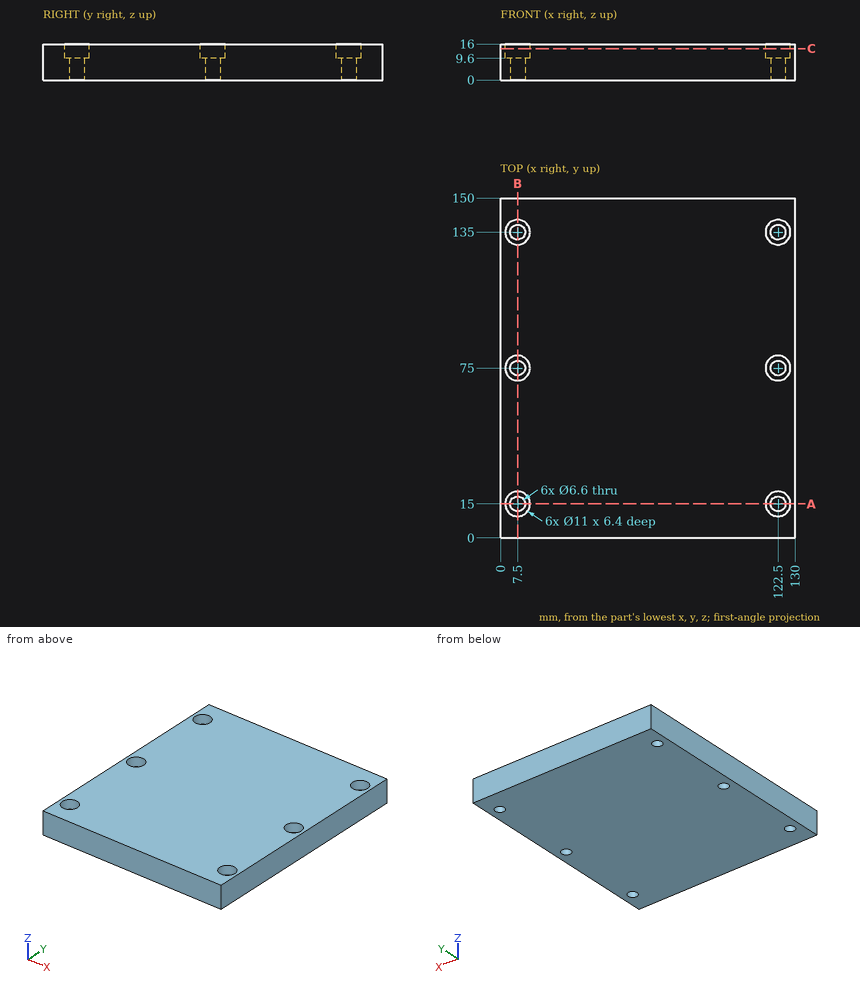
Can you work these out from the drawing? Everything is in mm from the part's minimum corner. Coordinates: 2 decimals unless noted, no trailing zeros. Order: outer loops, then holes, each group sorted by start corner. A loop starts at its lowest first (then second) coordinate and runs counter-clockwise, first axis right, second up. Notation, with made-up numbers: (52, 87) -> (107, 87) arc R18 cw to (107, 105) -> close; hole circle Ø9 at (68, -29). An arc over 180 degrees is marked (long way). Use one line per item in the form item = value.
Q1. I need wall thicknesses on L1, parallel to X at y = 135, z = 6.25; L2, parallel to Y at x = 7.5, z = 13; L3, parallel to X at y = 135, z = 14.75. Which ranges of each line are inside material? Lowest first, please.
From the geometry:
L1 = 0 to 4.2, 10.8 to 119.2, 125.8 to 130
L2 = 0 to 9.5, 20.5 to 69.5, 80.5 to 129.5, 140.5 to 150
L3 = 0 to 2, 13 to 117, 128 to 130
Q2. Imagine slicing it at C-C, the plane z = 14. List the corners of the cut face in (x, y) for me, then the cut area to 3 significant figures.
From the geometry:
outline = (0, 0) -> (130, 0) -> (130, 150) -> (0, 150) -> close; hole circle Ø11 at (7.5, 15); hole circle Ø11 at (7.5, 75); hole circle Ø11 at (7.5, 135); hole circle Ø11 at (122.5, 15); hole circle Ø11 at (122.5, 75); hole circle Ø11 at (122.5, 135)
area = 18,900 mm²
Q3. Imagine slicing it at A-A, the plane y = 15. List the corners of the cut face in (x, z) for me, then the cut area to 3 significant figures.
From the geometry:
outline = (0, 0) -> (4.2, 0) -> (4.2, 9.6) -> (2, 9.6) -> (2, 16) -> (0, 16) -> close; (10.8, 0) -> (119.2, 0) -> (119.2, 9.6) -> (117, 9.6) -> (117, 16) -> (13, 16) -> (13, 9.6) -> (10.8, 9.6) -> close; (125.8, 0) -> (130, 0) -> (130, 16) -> (128, 16) -> (128, 9.6) -> (125.8, 9.6) -> close
area = 1,810 mm²
Q4. Will this pin go through, and if not, where does the flat tip stop? P1, Ø10.5, axis at x = 122.5, y = 75, coming from the +Z side.
From the geometry:
P1 = 9.6
Q5. Imagine slicing it at B-B, the plane x = 7.5. List the corners of the cut face in (y, z) for me, then the cut area to 3 significant figures.
From the geometry:
outline = (0, 0) -> (11.7, 0) -> (11.7, 9.6) -> (9.5, 9.6) -> (9.5, 16) -> (0, 16) -> close; (18.3, 0) -> (71.7, 0) -> (71.7, 9.6) -> (69.5, 9.6) -> (69.5, 16) -> (20.5, 16) -> (20.5, 9.6) -> (18.3, 9.6) -> close; (78.3, 0) -> (131.7, 0) -> (131.7, 9.6) -> (129.5, 9.6) -> (129.5, 16) -> (80.5, 16) -> (80.5, 9.6) -> (78.3, 9.6) -> close; (138.3, 0) -> (150, 0) -> (150, 16) -> (140.5, 16) -> (140.5, 9.6) -> (138.3, 9.6) -> close
area = 2,000 mm²
